```python
from build123d import *

# Parameters (mm, degrees)
F0_W     = 25.4
F0_H     = 25.4
F1_DEPTH = 5.588
F3_T     = -2.54
F2_R     = 2.5146
F4_DEPTH = 1.905


with BuildPart() as f1:
    # F0 (on Front) → F1 (new body)
    with BuildSketch(Plane.XZ):
        Rectangle(F0_W, F0_H)
    extrude(amount=F1_DEPTH)

    # F3
    f3_openings = [f1.faces().sort_by_distance(p)[0] for p in [
        (0, 0, 0),
    ]]
    offset(amount=F3_T, openings=f3_openings)

    # F2 (on face) → F4 (join)
    with BuildSketch(Plane.XZ.offset(5.588)):
        with Locations((-7.9375, 7.9375)):
            Circle(F2_R)
        with Locations((0, 7.9375)):
            Circle(F2_R)
        with Locations((7.9375, 7.9375)):
            Circle(F2_R)
        with Locations((7.9375, 0)):
            Circle(F2_R)
        Circle(F2_R)
        with Locations((-7.9375, 0)):
            Circle(F2_R)
        with Locations((-7.9375, -7.9375)):
            Circle(F2_R)
        with Locations((0, -7.9375)):
            Circle(F2_R)
        with Locations((7.9375, -7.9375)):
            Circle(F2_R)
    extrude(amount=F4_DEPTH)


solid = f1.part
```
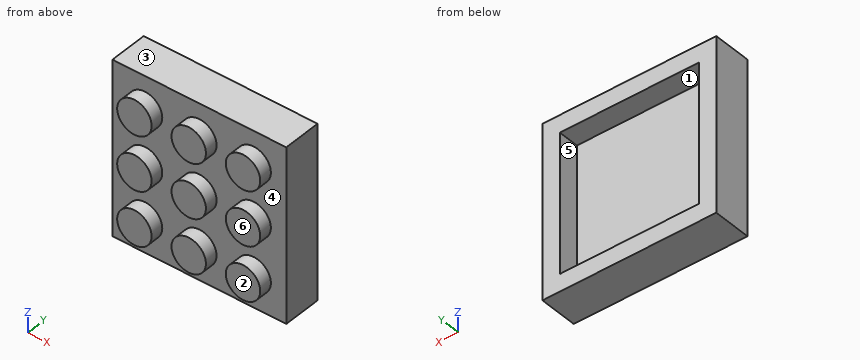
Check sheet for the modelled part. Datum: model origin and axes. Units: mm. Face numbers are marked on the shaded views. A direction names the side the tool comes from. Coordinates: 2 decimals unless noted, no trailing zeros. Order: outer loops, then holes, each group sorted by start corner. A loop starts at its lowest first (then second) coordinate and runs counter-clockwise, first axis right, second up. Notation, with made-up numbers: (-27.5, -2) -> (-3.5, -2) arc R13 ccw to (-3.5, 7) -> close; hole circle Ø7 at (72, -14.5). An arc over 180 degrees is marked (long way). Write each question's results on one line, items separated by ' | '. Start each with the question number.
1) Section check D-D (y = -6.5). Count the separate pieces of the cut face and the enclosed holes in it, and give its area (3 significant figures).
2) Draft check along Z on the marked faces 1, 2 and 3. Enter one of: pulls with the +Z half, pulls with the -Z half, needs draft (parallel to the pull), parting line crosses it, or undercut.
3) Section check A-A (y = -2.5). Enter the section's corners in (x, z).
4) Section check B-B (z = -4). Enter the section's corners in (x, y).
5) Section check C-C (x = 3). Enter the section's corners in (y, z).
6) Set-up check for the marked faces 4, 5 and 6: record each of +Z, -Z, +X, -X, +Y, -Y from which the full face is reachable in a straight line by a thin tool's end or side.
7) Depth check by flat-ended pin: pin 1 (6 mm diameter, centred on x = 4, z = 4, fed in from +Y). Enter the tip coordinate at first touch or a pass-through.
8) Material ranges on line 1 along X through (y, z) = (-1.75, -3.25); line 2 along Y through (x, z) = (6, 8), recorded low to high.
Checked values:
1) separate pieces: 9 | enclosed holes: 0 | area: 179 mm²
2) face 1: undercut | face 2: needs draft | face 3: pulls with the +Z half
3) outline: (-12.7, -12.7) -> (12.7, -12.7) -> (12.7, 12.7) -> (-12.7, 12.7) -> close; hole (-10.16, -10.16) -> (10.16, -10.16) -> (10.16, 10.16) -> (-10.16, 10.16) -> close
4) outline: (-12.7, -5.59) -> (12.7, -5.59) -> (12.7, 0) -> (10.16, 0) -> (10.16, -3.05) -> (-10.16, -3.05) -> (-10.16, 0) -> (-12.7, 0) -> close
5) outline: (-5.59, -12.7) -> (0, -12.7) -> (0, -10.16) -> (-3.05, -10.16) -> (-3.05, 10.16) -> (0, 10.16) -> (0, 12.7) -> (-5.59, 12.7) -> close
6) face 4: -Y | face 5: +Y | face 6: +Z, -Z, +X, -X, -Y
7) pin 1: y = -3.05
8) line 1: -12.7 to -10.16, 10.16 to 12.7 | line 2: -7.49 to -3.05
